Can you work these out from the model? Positions are in its coordinate system, mm. A direction names the side the tool comes from. Give positions to 0.01 mm unless a question says otherwise; leave off trailing zeros. Order: outer loops, then holes, each group sorted by start corner. A loop starts at its lowest first (then second) coordinate and runs counter-clockwise, first axis right, second up. Notation, with made-up numbers: (-33, 76.5) - (4, 76.5) arc R18 ccw to (4, 94.5) - close; hole circle Ø9 at (48, 30.25). An arc over 180 degrees is marked (long way). Return JSON: item names as keys, results as strings.
```python
from build123d import *

# Parameters (mm, degrees)
F1_DEPTH = 105
F2_R     = 2.1
F3_DEPTH = 87.001
F6_DEPTH = 2
F8_DEPTH = 2


with BuildPart() as f1:
    # F0 (on Front) → F1 (new body)
    with BuildSketch(Plane.XZ):
        with BuildLine():
            ThreePointArc((-41.5, 11.5), (-40.784767, 15.213907), (-38.741379, 18.396552))
            Line((-38.741379, 18.396552), (-42, 21.5))
            Line((-42, 21.5), (-42, 48.5))
            ThreePointArc((-42, 48.5), (-40.535534, 52.035534), (-37, 53.5))
            Line((-37, 53.5), (37, 53.5))
            ThreePointArc((37, 53.5), (40.535534, 52.035534), (42, 48.5))
            Line((42, 48.5), (42, 21.5))
            Line((42, 21.5), (38.741379, 18.396552))
            ThreePointArc((38.741379, 18.396552), (40.784767, 15.213907), (41.5, 11.5))
            Line((41.5, 11.5), (41.5, 5))
            Line((41.5, 5), (43.5, 5))
            Line((43.5, 5), (43.5, 49))
            ThreePointArc((43.5, 49), (41.742641, 53.242641), (37.5, 55))
            Line((37.5, 55), (-37.5, 55))
            ThreePointArc((-37.5, 55), (-41.742641, 53.242641), (-43.5, 49))
            Line((-43.5, 49), (-43.5, 5))
            Line((-43.5, 5), (-41.5, 5))
            Line((-41.5, 5), (-41.5, 11.5))
        make_face()
    extrude(amount=F1_DEPTH)

    # F2 (on face) → F3 (cut, through all)
    with BuildSketch(Plane.YZ.offset(43.5)):
        with Locations((-13.182085, 8)):
            Circle(F2_R)
    extrude(amount=-F3_DEPTH, mode=Mode.SUBTRACT)

    # F5 (on face) → F6 (join, symmetric)
    with BuildSketch(Plane.XZ.offset(105)):
        with BuildLine():
            Line((-42, 21.5), (-40, 21.5))
            Line((-40, 21.5), (-40, 47.5))
            ThreePointArc((-40, 47.5), (-38.828427, 50.328427), (-36, 51.5))
            Line((-36, 51.5), (36, 51.5))
            ThreePointArc((36, 51.5), (38.828427, 50.328427), (40, 47.5))
            Line((40, 47.5), (40, 21.5))
            Line((40, 21.5), (42, 21.5))
            Line((42, 21.5), (42, 48.5))
            ThreePointArc((42, 48.5), (40.535534, 52.035534), (37, 53.5))
            Line((37, 53.5), (-37, 53.5))
            ThreePointArc((-37, 53.5), (-40.535534, 52.035534), (-42, 48.5))
            Line((-42, 48.5), (-42, 21.5))
        make_face()
    extrude(amount=F6_DEPTH, both=True)

    # F7 (on face) → F8 (join, symmetric)
    with BuildSketch(Plane(origin=(0, 0, 0), x_dir=(-1, 0, 0), z_dir=(0, 1, 0))):
        with BuildLine():
            Line((-42, 48.5), (-42, 21.5))
            Line((-42, 21.5), (-40, 21.5))
            Line((-40, 21.5), (-40, 47.5))
            ThreePointArc((-40, 47.5), (-38.828427, 50.328427), (-36, 51.5))
            Line((-36, 51.5), (36, 51.5))
            ThreePointArc((36, 51.5), (38.828427, 50.328427), (40, 47.5))
            Line((40, 47.5), (40, 21.5))
            Line((40, 21.5), (42, 21.5))
            Line((42, 21.5), (42, 48.5))
            ThreePointArc((42, 48.5), (40.535534, 52.035534), (37, 53.5))
            Line((37, 53.5), (-37, 53.5))
            ThreePointArc((-37, 53.5), (-40.535534, 52.035534), (-42, 48.5))
        make_face()
    extrude(amount=F8_DEPTH, both=True)


solid = f1.part
```
1. Thinking about a two-plate mould opening in Y: for faces 5 (the face through (3, 2, 52)), 6 (the face through (42.51, -11.18, 8.63)), 7 (the face through (-40.57, 1.01, 52)), which applies, +Y half, -Y half, draft (parallel to the pull), parting line (faces both ways), or undercut?
Checks:
{"face 5": "+Y half", "face 6": "undercut", "face 7": "draft"}
2. For pin 1 Ø1.6 at (x, y) = (2, 1) entering from +Z; pin 2 Ø8 at (x, y) = (-10, -85.5) entering from -Z; pin 3 Ø0.6 at (y, z) = (-106, 40.5) entering from -X, each with a flat end and sliding along its axis, tell me the tip position at first contact or that it passes through.
Checks:
{"pin 1": "z = 53.5", "pin 2": "z = 53.5", "pin 3": "x = -42"}
3. Suppose I cut it at D-D (z = 8). List the corners of the cut face in (x, y) for me, plus the area to 3 significant figures.
Checks:
{"outline": "(-43.5, -105) - (-41.5, -105) - (-41.5, -15.28) - (-43.5, -15.28) - close; (-43.5, -11.08) - (-41.5, -11.08) - (-41.5, 0) - (-43.5, 0) - close; (41.5, -105) - (43.5, -105) - (43.5, -15.28) - (41.5, -15.28) - close; (41.5, -11.08) - (43.5, -11.08) - (43.5, 0) - (41.5, 0) - close", "area": "403 mm^2"}
4. Suppose I cut it at A-A (z = 43). List the corners of the cut face in (x, y) for me, plus the area to 3 significant figures.
Checks:
{"outline": "(-43.5, -105) - (-42, -105) - (-42, -107) - (-40, -107) - (-40, -103) - (-42, -103) - (-42, -2) - (-40, -2) - (-40, 2) - (-42, 2) - (-42, 0) - (-43.5, 0) - close; (40, -107) - (42, -107) - (42, -105) - (43.5, -105) - (43.5, 0) - (42, 0) - (42, 2) - (40, 2) - (40, -2) - (42, -2) - (42, -103) - (40, -103) - close", "area": "347 mm^2"}
5. Suppose I cut it at B-B (y = -59). List the corners of the cut face in (x, z) for me.
Checks:
{"outline": "(-43.5, 5) - (-41.5, 5) - (-41.5, 11.5) arc R10 cw to (-38.74, 18.4) - (-42, 21.5) - (-42, 48.5) arc R5 cw to (-37, 53.5) - (37, 53.5) arc R5 cw to (42, 48.5) - (42, 21.5) - (38.74, 18.4) arc R10 cw to (41.5, 11.5) - (41.5, 5) - (43.5, 5) - (43.5, 49) arc R6 ccw to (37.5, 55) - (-37.5, 55) arc R6 ccw to (-43.5, 49) - close"}
6. On a 3-axis mill with a long thin cutter (end or side, diameter ignored), from which of +Z, -Z, +X, -X, +Y, -Y can I reach the whole of each face in a straight line? I mean faces 1 (the face through (-1, -52, 53.5)), 2 (the face through (-41.5, -52, 8)), 3 (the face through (42, -52, 35)), 4 (the face through (40, 0, 34)). Say none if no direction works.
Checks:
{"face 1": "-Z", "face 2": "-Z, +Y, -Y", "face 3": "none", "face 4": "+Y, -Y"}
7. Suppose I cut it at C-C (x = -19). List the corners of the cut face in (y, z) for me.
Checks:
{"outline": "(-107, 51.5) - (-103, 51.5) - (-103, 53.5) - (-2, 53.5) - (-2, 51.5) - (2, 51.5) - (2, 53.5) - (0, 53.5) - (0, 55) - (-105, 55) - (-105, 53.5) - (-107, 53.5) - close"}
8. If I drill on L1, parallel to X at y = -3, z = 8; L2, parallel to X at y = -7, z = 34; L3, parallel to Y at x = -26.5, z = 52, over which ranges is the centre line in solid material (lowest first)? Write a range as [from, to].
Checks:
{"L1": "[-43.5, -41.5], [41.5, 43.5]", "L2": "[-43.5, -42], [42, 43.5]", "L3": "[-107, -103], [-2, 2]"}
